The listing builds one solid part. Answer for the finished solid, in the listing's coordinates (mm). A direction names the side the tool comes from. Coordinates: 2 decimals unless noted, no trailing zeros. Order: outer loops, then holes, each group sorted by start corner. A loop starts at its lowest first (then second) coordinate and runs counter-clockwise, first axis right, second up. Notation, with made-up numbers: (64, 88) - (101, 88) arc R23 cw to (101, 96) - close; hole circle Ø1 at (0, 45). An arc over 180 degrees is marked (long way). Use a Markdown table: item, result. Add a question column.
Item 1: For faces 1 (the flat face through (16.5, 4, -6)), 2 (the cylindrical face through (13.101, 3.698, -14.915)), 3 (the flat face through (-20, 4, 2.8)), determine the directions among +Z, -Z, +X, -X, +Y, -Y from which every point of the face is accessible in a straight line to the end or side of a thin tool.
Item 2: The mould has two halves that part along X. Classify faces 4 (the flat face through (-15, 4, -15.2)), 5 (the cylindrical face through (16.801, 3.698, 2.515)), 6 (the flat face through (12.8, 4, -8)): released by +X, released by -X, zero draft, split by the parting line, or undercut.
Item 3: The part is cut by section D-D, the plane z = 5.25. Give the vertices of the cut face in (x, y), then the cut area to 3 significant figures.
Item 4: Flat-ended cylindrical pins translate along their axes: P1, Ø4, axis at y = 5.5, z = -10, coming from the -X side; P2, Ø4, axis at x = -4.5, y = 3, coming from the -Z side; P3, Ø2, axis at x = 19, z = -3, coming from the -Y side (3 decimals); P4, Ø4, axis at y = 3, z = -11, coming from the +X side. Find the tip coordinate at first contact, or state that the pin passes through.
Item 5: The part is cut by section A-A, the plane z = -12.5. Give the vertices of the cut face in (x, y), then the cut area to 3 significant figures.
Item 6: The part is cut by section C-C, the plane y = 3.75. Give the vertices of the cut face in (x, z).
Item 7: The part is cut by section B-B, the plane x = 0. Give the vertices of the cut face in (y, z).
Item 8: Find the intervals of material crossed by line 1 along X through (y, z) = (3.75, 4); line 2 along X through (y, z) = (2.75, -5.75); line 3 along Y through (x, z) = (0, 5.5), in increasing order.
from build123d import *

# Parameters (mm, degrees)
BOSS_EXTRUDE1_DEPTH       = 7.5
BOSS_EXTRUDE2_DEPTH       = 7.5
FILLET1_R                 = 1
M6X1_0_TAPPED_HOLE1_D     = 5
M6X1_0_TAPPED_HOLE1_DEPTH = 9
M6X1_0_TAPPED_HOLE1_TIP   = 1.502151548


with BuildPart() as part:
    # Sketch1 → Boss-Extrude1 (new body)
    with BuildSketch(Plane(origin=(0, 0, 0), x_dir=(1, 0, 0), z_dir=(0, 1, 0))):
        with BuildLine():
            Line((-12, 0), (0, 0))
            Line((0, 0), (12, 0))
            Line((12, 0), (12, -2.8))
            Line((12, -2.8), (24, -2.8))
            Line((24, -2.8), (24, -8.576332159))
            ThreePointArc((24, -8.576332159), (0, -8), (-24, -8.576332159))
            Line((-24, -8.576332159), (-24, -2.8))
            Line((-24, -2.8), (-12, -2.8))
            Line((-12, -2.8), (-12, 0))
        make_face()
    extrude(amount=BOSS_EXTRUDE1_DEPTH)

    # Sketch5 → Boss-Extrude2 (add)
    with BuildSketch(Plane(origin=(0, 7.5, 0), x_dir=(1, 0, 0), z_dir=(0, 1, 0))):
        Polygon((12, 0), (12.8, 0), (12.8, 15.2), (16.5, 15.2), (16.5, -2.8), (12, -2.8), align=None)
        Polygon((-12, -2.8), (-12, 0), (-12.8, 0), (-12.8, 15.2), (-16.5, 15.2), (-16.5, -2.8), align=None)
    extrude(amount=-BOSS_EXTRUDE2_DEPTH)

    # Fillet1
    fillet1_edges = [part.edges().sort_by_distance(p)[0] for p in [
        (24, 3.75, 2.8),
        (-24, 3.75, 2.8),
        (16.5, 3.75, 2.8),
        (16.5, 3.75, -15.2),
        (12.8, 3.75, -15.2),
        (12.8, 3.75, 0),
        (-12.8, 3.75, 0),
        (-12.8, 3.75, -15.2),
        (-16.5, 3.75, -15.2),
        (-16.5, 3.75, 2.8),
    ]]
    fillet(fillet1_edges, radius=FILLET1_R)

    # M6x1.0 Tapped Hole1
    with Locations(Plane(origin=(0, 0, 0), x_dir=(-1, 0, 0), z_dir=(0, 0, -1))):
        with Locations((0, 3.75)):
            Hole(M6X1_0_TAPPED_HOLE1_D / 2, depth=M6X1_0_TAPPED_HOLE1_DEPTH)
            with Locations((0, 0, -(M6X1_0_TAPPED_HOLE1_DEPTH + M6X1_0_TAPPED_HOLE1_TIP / 2))):  # 118° drill point
                Cone(0, M6X1_0_TAPPED_HOLE1_D / 2, M6X1_0_TAPPED_HOLE1_TIP, mode=Mode.SUBTRACT)


solid = part.part
Solution:
| question | item | result |
|---|---|---|
| 1 | face 1 | -Z, +X, +Y, -Y |
| 1 | face 2 | -Z, +Y, -Y |
| 1 | face 3 | -Z, -X, +Y, -Y |
| 2 | face 4 | zero draft |
| 2 | face 5 | released by +X |
| 2 | face 6 | undercut |
| 3 | outline | (-24, 0) - (24, 0) - (24, 7.5) - (-24, 7.5) - close; hole circle Ø5 at (0, 3.75) |
| 3 | area | 340 mm2 |
| 4 | P1 | stops at x = -16.5 |
| 4 | P2 | stops at z = 0 |
| 4 | P3 | passes through |
| 4 | P4 | stops at x = 16.5 |
| 5 | outline | (-16.5, 0) - (-12.8, 0) - (-12.8, 7.5) - (-16.5, 7.5) - close; (12.8, 0) - (16.5, 0) - (16.5, 7.5) - (12.8, 7.5) - close |
| 5 | area | 55.5 mm2 |
| 6 | outline | (-24, 3.8) arc R1 ccw to (-23, 2.8) - (-17.5, 2.8) arc R1 cw to (-16.5, 1.8) - (-16.5, -14.2) arc R1 ccw to (-15.5, -15.2) - (-13.8, -15.2) arc R1 ccw to (-12.8, -14.2) - (-12.8, -1) arc R1 cw to (-11.8, 0) - (-2.5, 0) - (-2.5, 8.01) arc R500 cw to (-24, 8.58) - close; (2.5, 0) - (11.8, 0) arc R1 cw to (12.8, -1) - (12.8, -14.2) arc R1 ccw to (13.8, -15.2) - (15.5, -15.2) arc R1 ccw to (16.5, -14.2) - (16.5, 1.8) arc R1 cw to (17.5, 2.8) - (23, 2.8) arc R1 ccw to (24, 3.8) - (24, 8.58) arc R500 cw to (2.5, 8.01) - close |
| 7 | outline | (0, 0) - (1.25, 0) - (1.25, 8) - (0, 8) - close; (6.25, 0) - (7.5, 0) - (7.5, 8) - (6.25, 8) - close |
| 8 | line 1 | x = -24 to -2.5, 2.5 to 24 |
| 8 | line 2 | x = -16.5 to -12.8, 12.8 to 16.5 |
| 8 | line 3 | y = 0 to 1.25, 6.25 to 7.5 |
